Check sheet for the modelled part. Datum: model origin and axes. Units: mm. A direction names the side the tool comes from. Give positions to 0.01 mm unless a question says otherwise; leave off trailing zeros. Order: outer loops, then holes, each group sorted by start corner. A loop starts at its lowest first (then second) coordinate and runs counter-clockwise, first axis right, second up. Notation, with made-up numbers: (-37.5, -24.75) -> (4.5, -24.75) arc R7 ccw to (4.5, -20.75) -> close; hole circle Ø5 at (27, 6.25). An arc over 180 degrees is marked (long way). Write each question's results on one line, items separated by ' | '.
from build123d import *

# Parameters (mm, degrees)
BOSS_EXTRUDE2_DEPTH                          = 2
F_3_2_3_2_DIAMETER_HOLE3_D                   = 3.2
CSK_FOR_M3_FLAT_COUNTERSUNK_HEAD_SCR_2_COUNT = 2
CSK_FOR_M3_FLAT_COUNTERSUNK_HEAD_SCR_2_PITCH = 76
CSK_FOR_M3_FLAT_COUNTERSUNK_HEAD_SCR_3_COUNT = 2
CSK_FOR_M3_FLAT_COUNTERSUNK_HEAD_SCR_3_PITCH = 107.48023074
CSK_FOR_M3_FLAT_COUNTERSUNK_HEAD_SCR_4_COUNT = 2
CSK_FOR_M3_FLAT_COUNTERSUNK_HEAD_SCR_4_PITCH = 76
F_2_7_2_7_DIAMETER_HOLE1_D                   = 2.7
FILLET1_R                                    = 3
SKETCH26_W                                   = 6.5
SKETCH26_H                                   = 6.5
BOSS_EXTRUDE3_DEPTH                          = 2


with BuildPart() as part:
    # Sketch2 → Boss-Extrude2 (new body)
    with BuildSketch(Plane.ZY.offset(51.493641502)):
        Polygon((0.93465612, 3.45185693), (7.43465612, 3.45185693), (7.43465612, 86.45185693), (0.93465612, 86.45185693), (0.93465612, 92.95185693), (-82.06534388, 92.95185693), (-82.06534388, 86.45185693), (-88.56534388, 86.45185693), (-88.56534388, 3.45185693), (-82.06534388, 3.45185693), (-82.06534388, -3.04814307), (0.93465612, -3.04814307), align=None)
        Polygon((-82.06534388, 73.45185693), (-82.06534388, 16.45185693), (-69.06534388, 3.45185693), (-12.06534388, 3.45185693), (0.93465612, 16.45185693), (0.93465612, 73.45185693), (-12.06534388, 86.45185693), (-69.06534388, 86.45185693), align=None, mode=Mode.SUBTRACT)
    extrude(amount=BOSS_EXTRUDE2_DEPTH)

    # Ø3.2 (3.2) Diameter Hole3 (through all)
    with Locations(Plane.ZY.offset(53.493641502)):
        with Locations((-74.06534388, 0.20185693), (-85.31534388, 11.45185693), (-85.31534388, 78.45185693), (-74.06534388, 89.70185693), (-7.06534388, 89.70185693), (4.18465612, 78.45185693), (4.18465612, 11.45185693), (-7.06534388, 0.20185693)):
            Hole(F_3_2_3_2_DIAMETER_HOLE3_D / 2)

    # Sketch24 → CSK for M3 Flat Countersunk Head Screw5 (revolve, cut)
    with BuildSketch(Plane(origin=(-53.493641502, 6.95185693, -78.56534388), x_dir=(0, 0, 1), z_dir=(0, 1, 0))):
        Polygon((0, 0), (0, 2), (1.6, 2), (1.6, 1.65), (3.25, 0), align=None)
    csk_for_m3_flat_countersunk_head_screw5 = revolve(axis=Axis((-59.843641502, 6.95185693, -78.56534388), (1, 0, 0)), mode=Mode.SUBTRACT)

    # CSK for M3 Flat Countersunk Head Scr 2: CSK for M3 Flat Countersunk Head Screw5 ×2
    with Locations(*[(0, i * CSK_FOR_M3_FLAT_COUNTERSUNK_HEAD_SCR_2_PITCH, 0) for i in range(1, CSK_FOR_M3_FLAT_COUNTERSUNK_HEAD_SCR_2_COUNT)]):
        add(csk_for_m3_flat_countersunk_head_screw5, mode=Mode.SUBTRACT)

    # CSK for M3 Flat Countersunk Head Scr 3: CSK for M3 Flat Countersunk Head Screw5 ×2
    with Locations(*[Vector(0, 0.7071067811865478, 0.7071067811865472) * (i * CSK_FOR_M3_FLAT_COUNTERSUNK_HEAD_SCR_3_PITCH) for i in range(1, CSK_FOR_M3_FLAT_COUNTERSUNK_HEAD_SCR_3_COUNT)]):
        add(csk_for_m3_flat_countersunk_head_screw5, mode=Mode.SUBTRACT)

    # CSK for M3 Flat Countersunk Head Scr 4: CSK for M3 Flat Countersunk Head Screw5 ×2
    with Locations(*[(0, 0, i * CSK_FOR_M3_FLAT_COUNTERSUNK_HEAD_SCR_4_PITCH) for i in range(1, CSK_FOR_M3_FLAT_COUNTERSUNK_HEAD_SCR_4_COUNT)]):
        add(csk_for_m3_flat_countersunk_head_screw5, mode=Mode.SUBTRACT)

    # Ø2.7 (2.7) Diameter Hole1 (through all)
    with Locations(Plane(origin=(-53.493641502, 88.95185693, -65.56534388), x_dir=(0, 0, -1), z_dir=(-1, 0, 0))):
        with Locations((0, 0), (-50, 0), (0, 88), (-50, 88)):
            Hole(F_2_7_2_7_DIAMETER_HOLE1_D / 2)

    # Fillet1
    fillet1_edges = [part.edges().sort_by_distance(p)[0] for p in [
        (-52.493641502, 86.45185693, -69.06534388),
        (-52.493641502, 73.45185693, -82.06534388),
        (-52.493641502, 16.45185693, -82.06534388),
        (-52.493641502, 3.45185693, -69.06534388),
        (-52.493641502, 3.45185693, -12.06534388),
        (-52.493641502, 16.45185693, 0.93465612),
        (-52.493641502, 73.45185693, 0.93465612),
        (-52.493641502, 86.45185693, -12.06534388),
    ]]
    fillet(fillet1_edges, radius=FILLET1_R)

    # Sketch26 → Boss-Extrude3 (add)
    with BuildSketch(Plane(origin=(-51.493641502, 0, 0), x_dir=(0, 0, -1), z_dir=(1, 0, 0))):
        with Locations((-4.18465612, 89.70185693)):
            Rectangle(SKETCH26_W, SKETCH26_H)
        with Locations((85.31534388, 89.70185693)):
            Rectangle(SKETCH26_W, SKETCH26_H)
        with Locations((85.31534388, 0.20185693)):
            Rectangle(SKETCH26_W, SKETCH26_H)
        with Locations((-4.18465612, 0.20185693)):
            Rectangle(SKETCH26_W, SKETCH26_H)
    extrude(amount=-BOSS_EXTRUDE3_DEPTH)


solid = part.part
1. Section check A-A on y = 64. Record the cut outline in (x, z).
Verdict:
outline: (-53.49, -88.57) -> (-51.49, -88.57) -> (-51.49, -82.07) -> (-53.49, -82.07) -> close; (-53.49, 0.93) -> (-51.49, 0.93) -> (-51.49, 7.43) -> (-53.49, 7.43) -> close
2. Material ranges on probe 1 along Z at (x, y) = (-51.6, 46); probe 2 along Y at (x, z) = (-52.8, -28.5); probe 3 along Z at (x, y) = (-51.55, 6), recorded low to high. Write a range as from..to.
Verdict:
probe 1: z = -88.57..-82.07, 0.93..7.43 | probe 2: y = -3.05..3.45, 86.45..92.95 | probe 3: z = -88.57..-79.85, -77.28..-71.61, -9.52..-3.85, -1.28..7.43
3. Section check C-C on x = -53. Give the number of separate pieces and of enclosed holes in the cut face, then the cut area to 3 significant figures.
Verdict:
separate pieces: 1 | enclosed holes: 17 | area: 2,480 mm^2
4. Gauge pin test, flat end, axial feed: pin 1 Ø1.9 at (y, z) = (11.45, 4.18) entering from +X. Record the tip position at first contact, or that the pin passes through.
Verdict:
pin 1: passes through
5. Mould release check, pull along Z, two halves, no side actions. Record for faces 1 (the cylindrical face through (-52.48, 0.682, -75.591)), 2 (the cylindrical face through (-52, 91, -8)), 3 (the flat face through (-53.494, 46, -83)): +Z half, -Z half, draft (parallel to the pull), parting line (faces both ways), or undercut.
Verdict:
face 1: undercut | face 2: undercut | face 3: draft
6. Access from +Z, -Z, +X, -X, +Y, -Y to the whole of each face (thin tool, end or side, straight path). Record for faces 4 (the conical face through (-51.95, 7.99, -3.92)), 5 (the flat face through (-52.48, 10.031, -75.644)).
Verdict:
face 4: -X | face 5: +X, -X
7. Section check B-B on z = -41. Record the cut outline in (x, y).
Verdict:
outline: (-53.49, -3.05) -> (-51.49, -3.05) -> (-51.49, 3.45) -> (-53.49, 3.45) -> close; (-53.49, 86.45) -> (-51.49, 86.45) -> (-51.49, 92.95) -> (-53.49, 92.95) -> close
